For this review, take the finished solid that the model builds, in its own axes (mm). Face numbers are marked on the shaded views. A direction names the side the tool comes from. Give positions to 0.01 mm unless a question says otherwise; leave off trailing zeros. Loops run counter-clockwise (first coordinate to the right, second up) from the corner with the lowest first, then second, coordinate; pieces in that order, holes last.
```python
from build123d import *

# Parameters (mm, degrees)
BOSS_EXTRUDE1_DEPTH = 5


with BuildPart() as part:
    # Sketch1 → Boss-Extrude1 (new body)
    with BuildSketch(Plane(origin=(0, 0, 0), x_dir=(1, 0, 0), z_dir=(0, 1, 0))):
        with BuildLine():
            Line((1, 1.5), (1, 0.817081844))
            Line((1, 0.817081844), (2, 1.5))
            Line((2, 1.5), (3, 1.5))
            Line((3, 1.5), (3, -1.5))
            Line((3, -1.5), (-3, -1.5))
            Line((-3, -1.5), (-3, 1.5))
            Line((-3, 1.5), (-2, 1.5))
            Line((-2, 1.5), (-1, 0.817081844))
            Line((-1, 0.817081844), (-1, 1.5))
            Line((-1, 1.5), (-1, 2))
            ThreePointArc((-1, 2), (-1.146446609, 2.353553391), (-1.5, 2.5))
            Line((-1.5, 2.5), (-5, 2.5))
            Line((-5, 2.5), (-5, -2.5))
            Line((-5, -2.5), (5, -2.5))
            Line((5, -2.5), (5, 2.5))
            Line((5, 2.5), (1.5, 2.5))
            ThreePointArc((1.5, 2.5), (1.146446609, 2.353553391), (1, 2))
            Line((1, 2), (1, 1.5))
        make_face()
    extrude(amount=BOSS_EXTRUDE1_DEPTH)


solid = part.part
```
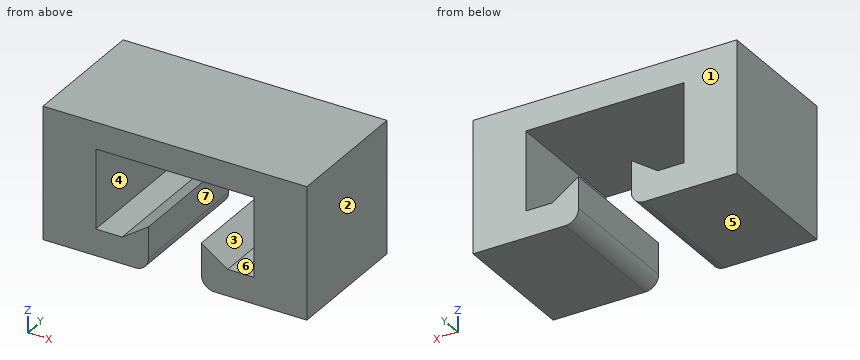
Q1. Mouldability with a two-part tool opening along X and no side actions: class the marked faces 1, 2, 3 and 4 as +X half, -X half, draft (parallel to the pull), parting line (faces both ways), or undercut.
Answers:
face 1: draft
face 2: +X half
face 3: undercut
face 4: undercut
Q2. Consider section B-B on x = 2.5. Give the boundary of the cut face in (y, z).
Answers:
outline: (0, -2.5) - (5, -2.5) - (5, -1.5) - (0, -1.5) - close; (0, 1.5) - (5, 1.5) - (5, 2.5) - (0, 2.5) - close
Q3. Consider section A-A on z = -1.85. Give the boundary of the cut face in (x, y).
Answers:
outline: (-5, 0) - (-1, 0) - (-1, 5) - (-5, 5) - close; (1, 0) - (5, 0) - (5, 5) - (1, 5) - close
Q4. Consider section C-C on y = 0.45. Give the boundary of the cut face in (x, z).
Answers:
outline: (-5, -2.5) - (-1.5, -2.5) arc R0.5 ccw to (-1, -2) - (-1, -0.82) - (-2, -1.5) - (-3, -1.5) - (-3, 1.5) - (3, 1.5) - (3, -1.5) - (2, -1.5) - (1, -0.82) - (1, -2) arc R0.5 ccw to (1.5, -2.5) - (5, -2.5) - (5, 2.5) - (-5, 2.5) - close
Q5. For probe 1 along X at (y, z) = (0.4, -1.55); probe 2 along X at (y, z) = (3.05, 0.75); probe 3 along Z at (x, y) = (-2.5, 1.7), list the stretches that pass through material, from the lowest coordinate up.
Answers:
probe 1: x = -5 to -1, 1 to 5
probe 2: x = -5 to -3, 3 to 5
probe 3: z = -2.5 to -1.5, 1.5 to 2.5
Q6. Consider section D-D on x = 0. Give the boundary of the cut face in (y, z).
Answers:
outline: (0, 1.5) - (5, 1.5) - (5, 2.5) - (0, 2.5) - close
Q7. Machinability: for the marked faces 5, 6 and 7, which of the approach directions +Z, -Z, +X, -X, +Y, -Y give a long, thin tool a straight path to every point of the face, cutting with its end or side? Answer none if there is none.
Answers:
face 5: -Z, +X, -X, +Y, -Y
face 6: +Y, -Y
face 7: -Z, +Y, -Y
